from build123d import *

# Parameters (mm, degrees)
SKETCH1_W                 = 10.42
SKETCH1_H                 = 2.5
BOSS_EXTRUDE1_DEPTH       = 6.2
SKETCH2_W                 = 2.04
SKETCH2_H                 = 1.5
CUT_EXTRUDE1_DEPTH        = 5.7
SKETCH3_W                 = 1.6
SKETCH3_H                 = 1.6
CUT_EXTRUDE2_DEPTH        = 0.5
CUT_EXTRUDE2_DRAFT        = -45
LPATTERN1_COUNT           = 4
LPATTERN1_PITCH           = 2.54
LPATTERN1_COPY_1_SKETCH_W = 1.6
LPATTERN1_COPY_1_SKETCH_H = 1.6
LPATTERN1_COPY_1_DEPTH    = 0.5
LPATTERN1_COPY_1_DRAFT    = -45
LPATTERN1_COPY_2_SKETCH_W = 1.6
LPATTERN1_COPY_2_SKETCH_H = 1.6
LPATTERN1_COPY_2_DEPTH    = 0.5
LPATTERN1_COPY_2_DRAFT    = -45
LPATTERN1_COPY_3_SKETCH_W = 1.6
LPATTERN1_COPY_3_SKETCH_H = 1.6
LPATTERN1_COPY_3_DEPTH    = 0.5
LPATTERN1_COPY_3_DRAFT    = -45
SKETCH4_W                 = 10.42
SKETCH4_H                 = 0.5
BOSS_EXTRUDE2_DEPTH       = 0.1


with BuildPart() as part:
    # Sketch1 → Boss-Extrude1 (new body)
    with BuildSketch(Plane(origin=(0, 0, 0), x_dir=(1, 0, 0), z_dir=(0, 1, 0))):
        Rectangle(SKETCH1_W, SKETCH1_H)
    extrude(amount=BOSS_EXTRUDE1_DEPTH)

    # Sketch2 → Cut-Extrude1 (cut)
    with BuildSketch(Plane(origin=(0, 6.2, 0), x_dir=(1, 0, 0), z_dir=(0, 1, 0))):
        with Locations((-3.81, 0)):
            Rectangle(SKETCH2_W, SKETCH2_H)
    cut_extrude1 = extrude(amount=-CUT_EXTRUDE1_DEPTH, mode=Mode.SUBTRACT)


with BuildPart() as cut_extrude2_tool:
    # Sketch3 → Cut-Extrude2 (with draft: the straight prism first)
    with BuildSketch(Plane.XZ):
        with Locations((-3.81, 0)):
            Rectangle(SKETCH3_W, SKETCH3_H)
    extrude(amount=-CUT_EXTRUDE2_DEPTH)
    # Cut-Extrude2: the draft: its side faces are tilted about the plane it starts from
    cut_extrude2_sides = [cut_extrude2_tool.faces().sort_by_distance(p)[0] for p in [
        (-3.81, 0.25, -0.8),
        (-3.01, 0.25, 0),
        (-3.81, 0.25, 0.8),
        (-4.61, 0.25, 0),
    ]]
    draft(cut_extrude2_sides, Plane.XZ, CUT_EXTRUDE2_DRAFT)


with BuildPart() as part_1:
    add(part.part)

    # Cut-Extrude2: cut by cut_extrude2_tool
    add(cut_extrude2_tool.part, mode=Mode.SUBTRACT)

    # LPattern1: Cut-Extrude1 ×4
    with Locations(*[(i * LPATTERN1_PITCH, 0, 0) for i in range(1, LPATTERN1_COUNT)]):
        add(cut_extrude1, mode=Mode.SUBTRACT)


with BuildPart() as lpattern1_copy_1_tool:
    # LPattern1 copy 1 sketch → LPattern1 copy 1 (with draft: the straight prism first)
    with BuildSketch(Plane(origin=(2.54, 0, 0), x_dir=(1, 0, 0), z_dir=(0, -1, 0))):
        with Locations((-3.81, 0)):
            Rectangle(LPATTERN1_COPY_1_SKETCH_W, LPATTERN1_COPY_1_SKETCH_H)
    extrude(amount=-LPATTERN1_COPY_1_DEPTH)
    # LPattern1 copy 1: the draft: its side faces are tilted about the plane it starts from
    lpattern1_copy_1_sides = [lpattern1_copy_1_tool.faces().sort_by_distance(p)[0] for p in [
        (-1.27, 0.25, -0.8),
        (-0.47, 0.25, 0),
        (-1.27, 0.25, 0.8),
        (-2.07, 0.25, 0),
    ]]
    draft(lpattern1_copy_1_sides, Plane(origin=(2.54, 0, 0), x_dir=(1, 0, 0), z_dir=(0, -1, 0)), LPATTERN1_COPY_1_DRAFT)


with BuildPart() as part_2:
    add(part_1.part)

    # LPattern1 copy 1: cut by lpattern1_copy_1_tool
    add(lpattern1_copy_1_tool.part, mode=Mode.SUBTRACT)


with BuildPart() as lpattern1_copy_2_tool:
    # LPattern1 copy 2 sketch → LPattern1 copy 2 (with draft: the straight prism first)
    with BuildSketch(Plane(origin=(5.08, 0, 0), x_dir=(1, 0, 0), z_dir=(0, -1, 0))):
        with Locations((-3.81, 0)):
            Rectangle(LPATTERN1_COPY_2_SKETCH_W, LPATTERN1_COPY_2_SKETCH_H)
    extrude(amount=-LPATTERN1_COPY_2_DEPTH)
    # LPattern1 copy 2: the draft: its side faces are tilted about the plane it starts from
    lpattern1_copy_2_sides = [lpattern1_copy_2_tool.faces().sort_by_distance(p)[0] for p in [
        (1.27, 0.25, -0.8),
        (2.07, 0.25, 0),
        (1.27, 0.25, 0.8),
        (0.47, 0.25, 0),
    ]]
    draft(lpattern1_copy_2_sides, Plane(origin=(5.08, 0, 0), x_dir=(1, 0, 0), z_dir=(0, -1, 0)), LPATTERN1_COPY_2_DRAFT)


with BuildPart() as part_3:
    add(part_2.part)

    # LPattern1 copy 2: cut by lpattern1_copy_2_tool
    add(lpattern1_copy_2_tool.part, mode=Mode.SUBTRACT)


with BuildPart() as lpattern1_copy_3_tool:
    # LPattern1 copy 3 sketch → LPattern1 copy 3 (with draft: the straight prism first)
    with BuildSketch(Plane(origin=(7.62, 0, 0), x_dir=(1, 0, 0), z_dir=(0, -1, 0))):
        with Locations((-3.81, 0)):
            Rectangle(LPATTERN1_COPY_3_SKETCH_W, LPATTERN1_COPY_3_SKETCH_H)
    extrude(amount=-LPATTERN1_COPY_3_DEPTH)
    # LPattern1 copy 3: the draft: its side faces are tilted about the plane it starts from
    lpattern1_copy_3_sides = [lpattern1_copy_3_tool.faces().sort_by_distance(p)[0] for p in [
        (3.81, 0.25, -0.8),
        (4.61, 0.25, 0),
        (3.81, 0.25, 0.8),
        (3.01, 0.25, 0),
    ]]
    draft(lpattern1_copy_3_sides, Plane(origin=(7.62, 0, 0), x_dir=(1, 0, 0), z_dir=(0, -1, 0)), LPATTERN1_COPY_3_DRAFT)


with BuildPart() as part_4:
    add(part_3.part)

    # LPattern1 copy 3: cut by lpattern1_copy_3_tool
    add(lpattern1_copy_3_tool.part, mode=Mode.SUBTRACT)

    # Sketch4 → Boss-Extrude2 (add)
    with BuildSketch(Plane(origin=(0, 6.2, 0), x_dir=(1, 0, 0), z_dir=(0, 1, 0))):
        with Locations((0, 1)):
            Rectangle(SKETCH4_W, SKETCH4_H)
    boss_extrude2 = extrude(amount=BOSS_EXTRUDE2_DEPTH)

    # Mirror1: Boss-Extrude2 across plane
    add(boss_extrude2.mirror(Plane.XY))


solid = part_4.part
Build history of the part. All positions in model axes, mm. A direction names the side the tool comes from. Coordinates: 2 decimals unless noted, no trailing zeros. Write each loop counter-clockwise with the first axis right and the second up, starting at its lowest first coordinate (ties: lowest second). Pieces come first, ordered by that corner, then holes.
(1) 3-axis set-ups, long thin cutter, end or side, ignore diameter. For faces 4 (the flat face through (-5.21, 3, 0)), 5 (the flat face through (-2.79, 3, 0)): which of +Z, -Z, +X, -X, +Y, -Y reach the whole face in a straight line?
(2) Cut at A-A on x = 3.75. List the corners of the cut face in (y, z).
(3) Pin check, flat tips, straight feed: pin 1 Ø0.8 at (x, z) = (3.5, 0) entering from +Y; pin 2 Ø1.5 at (x, z) = (-3, -0.5) entering from +Y; pin 3 Ø0.6 at (x, z) = (-2.5, 0) entering from +Y. Stop position of each tip, or through.
(4) Drill centre lines: line 1 (X direction, y = 4, z = -0.7); line 2 (Z direction, x = 4, y = 3.75); line 3 (Y direction, x = -2.5, z = 0.2). Where is each one in solid material? Low to high.
(5) Cut at B-B on y = 3. List the corners of the cut face in (x, z).
(6) Cut at C-C on z = -0.2. State how many separate pieces and enclosed holes the cut face has, and give its area (3 significant figures).
(7) Mould opens along X. For faces 1 (the flat face through (0, 3, 1.25)), 2 (the flat face through (2.79, 3, 0)), 3 (the flat face through (5.21, 3, 0)) say: pulls with the +X half, pulls with the -X half, needs draft (parallel to the pull), parting line crosses it, or undercut.
Working result:
1. face 4: +Z, -Z, -X, +Y, -Y
1. face 5: +Y
2. outline: (0, -1.25) - (6.3, -1.25) - (6.3, -0.75) - (0.5, -0.75) - (0.5, -0.3) - (0, -0.8) - close; (0, 0.8) - (0.5, 0.3) - (0.5, 0.75) - (6.3, 0.75) - (6.3, 1.25) - (0, 1.25) - close
3. pin 1: stops at y = 0.5
3. pin 2: stops at y = 6.3
3. pin 3: stops at y = 6.2
4. line 1: x = -5.21 to -4.83, -2.79 to -2.29, -0.25 to 0.25, 2.29 to 2.79, 4.83 to 5.21
4. line 2: z = -1.25 to -0.75, 0.75 to 1.25
4. line 3: y = 0 to 6.2
5. outline: (-5.21, -1.25) - (5.21, -1.25) - (5.21, 1.25) - (-5.21, 1.25) - close; hole (-4.83, -0.75) - (-2.79, -0.75) - (-2.79, 0.75) - (-4.83, 0.75) - close; hole (-2.29, -0.75) - (-0.25, -0.75) - (-0.25, 0.75) - (-2.29, 0.75) - close; hole (0.25, -0.75) - (2.29, -0.75) - (2.29, 0.75) - (0.25, 0.75) - close; hole (2.79, -0.75) - (4.83, -0.75) - (4.83, 0.75) - (2.79, 0.75) - close
6. separate pieces: 5
6. enclosed holes: 0
6. area: 15.9 mm2
7. face 1: needs draft
7. face 2: undercut
7. face 3: pulls with the +X half
